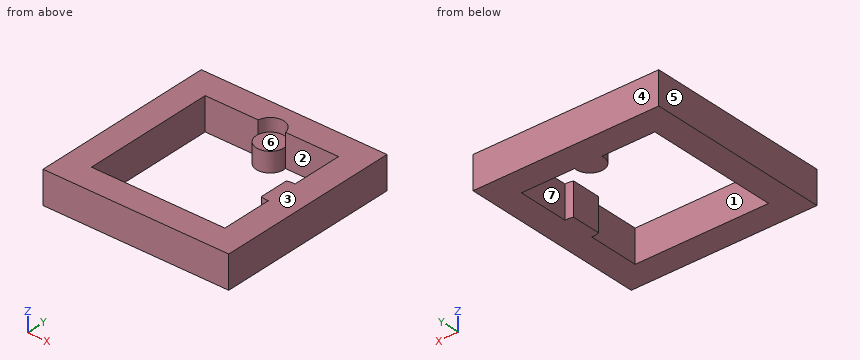
Autodesk Fusion 360 part; units mm, degrees
sketch "Sketch1" plane through (0, 0, 0) normal (0, 0, 1) x (1, 0, 0)
  line L0 (14.2, -14.2) -> (-14.2, -14.2)
  line L1 (-14.2, -14.2) -> (-14.2, 14.2)
  line L2 (-14.2, 14.2) -> (14.2, 14.2)
  line L3 (14.2, 14.2) -> (14.2, -14.2)
  line L4 (14.2, -14.2) -> (-14.2, 14.2) construction
  line L5 (-14.2, -14.2) -> (14.2, 14.2) construction
  dimension "d1" = 28.4
  dimension "d2" = 28.4
extrude "Extrude1" add sketch "Sketch1" along normal blind 5
shell "Shell1" thickness 4 removed faces 2 at (-4.7333, 4.7333, 5) at (-4.7333, 4.7333, 0)
sketch "Sketch2" plane through (0, 0, 5) normal (0, 0, 1) x (-1, 0, 0)
  line L0 (-10.2, -10.2) -> (-10.2, 10.2)
  line L1 (-10.2, 10.2) -> (10.2, 10.2)
  line L2 (10.2, 10.2) -> (10.2, -10.2)
  line L3 (10.2, -10.2) -> (-10.2, -10.2)
  line L4 (-14.2, -14.2) -> (14.2, -14.2)
  line L5 (14.2, -14.2) -> (14.2, 14.2)
  line L6 (14.2, 14.2) -> (-14.2, 14.2)
  line L7 (-14.2, 14.2) -> (-14.2, -14.2)
  circle A0 centre (0, -9.9) radius 2.1
  circle A1 centre (-9.9, 0) radius 2.4
  line L8 (-10.2, 0) -> (10.2, 0) construction
  line L9 (0, -10.2) -> (0, 10.2) construction
  circle A2 centre (0, 9.9) radius 2.1
  circle A3 centre (9.9, 0) radius 2.4
  line L10 (-9, -2.2249) -> (-9, 2.2249)
  dimension "d11" = 4.2
  dimension "d12" = 0.3
  dimension "d14" = 4.8
  dimension "d15" = 0.3
  dimension "d18" = 4.2
  dimension "d19" = 0.3
  dimension "d21" = 4.8
  dimension "d31" = 0.3
  dimension "d33" = 0.9
extrude "Extrude2" add sketch "Sketch2" against normal blind 5 contours L0 A1 L10 | L2 A3 picked at (10.826, 0.3361)
extrude "Extrude3" cut sketch "Sketch2" against normal blind 2 contours L3 A0 | L1 A2 picked at (0.357, -10.7865) picked at (0.2572, 9.449)
extrude "Extrude4" add sketch "Sketch2" against normal blind 3 from surface at -2 contours L3 A0 | L1 A2 picked at (0.2572, -9.449) picked at (0.0996, 10.7929)
The listing builds one solid part. Answer for the finished solid, in the listing's coordinates (mm). Face numbers are marked on the shaded views. A direction names the side the tool comes from. Round coordinates to 2 decimals unless told otherwise and drop trailing zeros. Order: outer loops, then holes, each group sorted by start corner. A loop starts at its lowest first (then second) coordinate and runs counter-clockwise, first axis right, second up. Notation, with made-up numbers: (33, -36.75) -> (78, -36.75) arc R15 cw to (78, -32.75) -> close; hole circle Ø3 at (46, -29.5). An arc over 180 degrees is marked (long way). Answer as CSV lines item,"result". Start each with the question number.
(1) Find the intervals of material crossed by probe 1 along X at (y, z) = (10, 1.5); probe 2 along Y at (x, z) = (-9.75, 4.7), in increasing order. Write a range as from..to.
(2) The part is cut by section C-C (x = 9.75). Determine the outline of the cut face in (y, z).
(3) For a pull along Y with two mould halves and no side action, classify the marked faces 1, 2, 3 and 4 as +Y half, -Y half, draft (parallel to the pull), parting line (faces both ways), or undercut.
(4) A tool of negligible diameter and unlimited length cuts with its end or side. For the marked faces 5, 6 and 7, from which of +Z, -Z, +X, -X, +Y, -Y can it reach the whole face along a straight path? Write none if from no direction.
(5) The part is cut by section D-D (z = 4.3). Determine the outline of the cut face in (x, y), then the cut area to 3 significant figures.
(6) A flat-ended cylindrical pin translates along its axis: pin 1 Ø3.5 at (x, y) = (0, 9) entering from +Z. Find the tip coordinate at first contact, or state that the pin passes through.
(7) The part is cut by section A-A (x = 6.25). Determine the outline of the cut face in (y, z).
Evaluation:
1,probe 1,"-14.2..-10.2, -2.1..2.1, 10.2..14.2"
1,probe 2,"-14.2..-10.2, 10.2..14.2"
2,outline,"(-14.2, 0) -> (-10.2, 0) -> (-10.2, 5) -> (-14.2, 5) -> close; (-2.4, 0) -> (2.4, 0) -> (2.4, 5) -> (-2.4, 5) -> close; (10.2, 0) -> (14.2, 0) -> (14.2, 5) -> (10.2, 5) -> close"
3,face 1,"undercut"
3,face 2,"undercut"
3,face 3,"draft"
3,face 4,"+Y half"
4,face 5,"+Z, -Z, -X, +Y, -Y"
4,face 6,"+Z"
4,face 7,"+Z, -Z"
5,outline,"(-14.2, -14.2) -> (14.2, -14.2) -> (14.2, 14.2) -> (-14.2, 14.2) -> close; hole (-10.2, -10.2) -> (10.2, -10.2) -> (10.2, -2.38) arc R2.4 cw to (9, -2.22) -> (9, 2.22) arc R2.4 cw to (10.2, 2.38) -> (10.2, 10.2) -> (2.08, 10.2) arc R2.1 ccw to (-2.08, 10.2) -> (-10.2, 10.2) -> close"
5,area,"390 mm²"
6,pin 1,"z = 3"
7,outline,"(-14.2, 0) -> (-10.2, 0) -> (-10.2, 5) -> (-14.2, 5) -> close; (10.2, 0) -> (14.2, 0) -> (14.2, 5) -> (10.2, 5) -> close"
